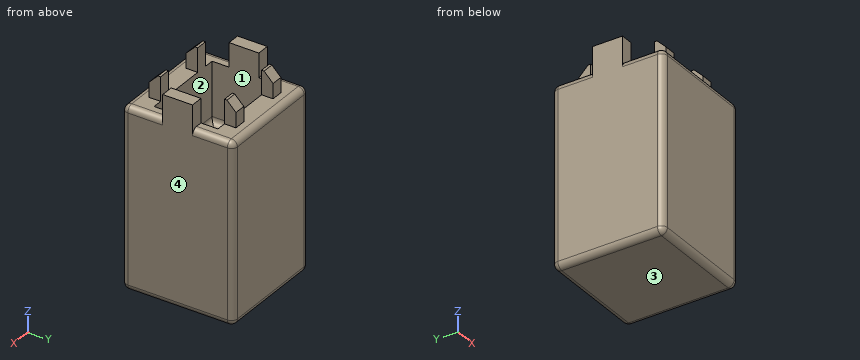
Autodesk Fusion 360 part; units mm, degrees
sketch "Sketch1" plane through (0, 0, 0) normal (0, 0, 1) x (1, 0, 0)
  line L0 (0, 0) -> (18.62, 0)
  line L1 (18.62, 0) -> (18.62, 14.49)
  line L2 (18.62, 14.49) -> (0, 14.49)
  line L3 (0, 14.49) -> (0, 0)
  line L4 (9.31, 0) -> (9.31, 14.49)
  line L5 (0, 7.245) -> (18.62, 7.245)
  line L6 (2.1, 9.73) -> (-2.1, 9.73)
  line L7 (-2.1, 9.73) -> (-2.1, 4.76)
  line L8 (-2.1, 4.76) -> (2.1, 4.76)
  line L9 (2.1, 4.76) -> (2.1, 9.73)
  line L10 (2.1, 9.73) -> (-2.1, 4.76) construction
  line L11 (-2.1, 9.73) -> (2.1, 4.76) construction
  line L12 (3.72, 0) -> (3.72, 14.49)
  line L13 (3.72, 14.49) -> (5.66, 14.49)
  line L14 (5.66, 14.49) -> (5.66, 12.57)
  line L15 (5.66, 12.57) -> (3.72, 12.57)
  line L16 (3.72, 12.57) -> (3.72, 14.49)
  line L17 (5.66, 1.92) -> (3.72, 1.92)
  line L18 (3.72, 1.92) -> (3.72, 0)
  line L19 (5.66, 0) -> (5.66, 1.92)
  line L20 (16.52, 9.73) -> (20.72, 9.73)
  line L21 (16.52, 4.76) -> (16.52, 9.73)
  line L22 (20.72, 4.76) -> (16.52, 4.76)
  line L23 (12.96, 14.49) -> (12.96, 12.57)
  line L24 (12.96, 12.57) -> (14.9, 12.57)
  line L25 (14.9, 12.57) -> (14.9, 14.49)
  line L26 (12.96, 1.92) -> (14.9, 1.92)
  line L27 (12.96, 0) -> (12.96, 1.92)
  line L28 (14.9, 0) -> (14.9, 14.49)
  line L29 (3.72, 12.57) -> (14.9, 12.57)
  line L30 (14.9, 12.57) -> (14.9, 1.92)
  line L31 (14.9, 1.92) -> (3.72, 1.92)
  line L32 (3.72, 1.92) -> (3.72, 12.57)
  line L33 (2.1, 9.73) -> (3.72, 9.73)
  line L34 (3.72, 9.73) -> (3.72, 12.57)
  line L35 (3.72, 12.57) -> (2.1, 12.57)
  line L36 (2.1, 12.57) -> (2.1, 9.73)
  line L37 (2.1, 4.76) -> (3.72, 4.76)
  line L38 (3.72, 4.76) -> (3.72, 1.92)
  line L39 (3.72, 1.92) -> (2.1, 1.92)
  line L40 (2.1, 1.92) -> (2.1, 4.76)
  line L41 (14.9, 1.92) -> (16.52, 1.92)
  line L42 (16.52, 1.92) -> (16.52, 4.76)
  line L43 (16.52, 4.76) -> (14.9, 4.76)
  line L44 (14.9, 4.76) -> (14.9, 1.92)
  line L45 (16.52, 9.73) -> (14.9, 9.73)
  line L46 (14.9, 9.73) -> (14.9, 12.57)
  line L47 (14.9, 12.57) -> (16.52, 12.57)
  line L48 (16.52, 12.57) -> (16.52, 9.73)
  circle A0 centre (9.31, 7.245) radius 2.5
  line L49 (18.62, -2.065) -> (0, -2.065)
  line L50 (0, -2.065) -> (0, 16.555)
  line L51 (0, 16.555) -> (18.62, 16.555)
  line L52 (18.62, 16.555) -> (18.62, -2.065)
  line L53 (18.62, -2.065) -> (0, 16.555) construction
  line L54 (0, -2.065) -> (18.62, 16.555) construction
  point P0 (0, 7.245)
  point P1 (9.31, 7.245)
  dimension "d1" = 18.62
  dimension "d2" = 14.49
  dimension "d3" = 4.2
  dimension "d4" = 4.97
  dimension "d5" = -5.59
  dimension "d6" = 1.94
  dimension "d7" = 1.92
  dimension "d16" = 5
  dimension "d19" = 18.62
  dimension "d20" = 18.62
extrude "Extrude1" add sketch "Sketch1" along normal blind 34 contours L0 L12 L17 L18 L19 L31 | L3 L5 L8 L9 L50 | L3 L5 L6 L9 L50 | L0 L26 L27 L28 L31 | L1 L5 L21 L22 L52 | L2 L12 L13 L14 L15 L16 L29 | L1 L5 L20 L21 L52 | L2 L23 L24 L25 L28 L29 makes body 1 at (13.6067, 0, 22.6667) makes body 2 at (5.0133, 14.49, 22.6667) makes body 3 at (18.62, 6.4167, 11.3333) makes body 4 at (4.3667, 0, 22.6667) makes body 5 at (0, 8.0733, 11.3333) makes body 6 at (14.2533, 14.49, 22.6667)
extrude "Extrude4" add sketch "Sketch1" along normal blind 30 contours L0 L3 L8 L12 L18 L39 L40 L50 | L0 L4 L19 L31 | L0 L4 L27 L31 | L2 L3 L6 L12 L16 L35 L36 L50 | L0 L1 L22 L28 L41 L42 L52 | L2 L4 L14 L29 | L1 L2 L20 L25 L28 L47 L48 L52 | L2 L4 L23 L29 bodies 1 2 3 4 5 6
extrude "Extrude5" add sketch "Sketch1" along normal blind 20 contours L12 L32 L37 L38 L39 L40 | L4 L5 L12 L17 L31 L32 L38 A0 | L5 L9 L12 L32 L37 | L5 L9 L12 L32 L33 | L4 L5 L26 L28 L30 L31 L44 A0 | L4 L5 L12 L15 L29 L32 L34 A0 | L12 L32 L33 L34 L35 L36 | L4 L5 A0 | L4 L5 A0 | L4 L5 A0 | L28 L30 L41 L42 L43 L44 | L5 L21 L28 L30 L43 | L4 L5 A0 | L4 L5 L24 L28 L29 L30 L46 A0 | L5 L21 L28 L30 L45 | L28 L30 L45 L46 L47 L48 bodies 1
extrude "Extrude6" add sketch "Sketch1" along normal blind 30 contours L0 L49 L50 L52 | L2 L13 L50 L51 L52 bodies 1
fillet "Fillet1" radius 1 4 edges at (18.62, 16.555, 15) (0, 16.555, 15) (0, -2.065, 15) (18.62, -2.065, 15) on bodies 1
fillet "Fillet2" radius 1 10 edges at (18.62, 12.6425, 30) (18.3271, 16.2621, 30) (9.31, 16.555, 30) (0.2929, 16.2621, 30) (0, 12.6425, 30) (0, 1.8475, 30) (0.2929, -1.7721, 30) (9.31, -2.065, 30) (18.3271, -1.7721, 30) (18.62, 1.8475, 30) on bodies 1
chamfer "Chamfer1" distance 1.5 angle 45 1 edges at (4.69, 0, 34) on bodies 1
chamfer "Chamfer2" distance 1.5 angle 45 1 edges at (13.93, 0, 34) on bodies 1
chamfer "Chamfer3" distance 1.5 angle 45 2 edges at (4.69, 14.49, 34) (13.93, 14.49, 34) on bodies 1
fillet "Fillet3" radius 1 4 edges at (9.31, 1.92, 20) (16.52, 7.245, 20) (2.1, 7.245, 20) (9.31, 12.57, 20) on bodies 1
fillet "Fillet4" radius 1 8 edges at (0.2929, -1.7721, 0) (0, 7.245, 0) (0.2929, 16.2621, 0) (9.31, 16.555, 0) (18.3271, 16.2621, 0) (18.62, 7.245, 0) (18.3271, -1.7721, 0) (9.31, -2.065, 0) on bodies 1
scale "Scale1" factor 1.01 about (0, -1.065, 29) bodies 1
Source: CAD feature listing. Evaluate the final solid. Frame: model axes, mm. Face numbers are marked on the shaded views. Round coordinates to 2 decimals unless told otherwise and drop trailing zeros. Loops run counter-clockwise (first coordinate to the right, second up) from the corner with the lowest first, then second, coordinate; pieces in that order, holes last. Notation, with made-up numbers: (-8.75, 57.25) -> (10.25, 57.25) arc R26 ccw to (10.25, 87.25) -> close; hole circle Ø2 at (-17, -7). An arc over 180 degrees is marked (long way). Answer as a JSON object with one key per item and string values. Group by question number.
Q1. Section query C-C (x = 17.25). Output: boundary loops of the cut face in (y, z) (3 decimals), plus the area to 3 significant figures.
Q2. Contact query for flat-ended pins moving along their axis: P1, Ø1, axis at y = 14, z = 32, coming from the +X side; P2, Ø0.6, axis at x = 17.5, z = 32, coming from the -Y side; P3, Ø1, axis at y = 1, z = 32, coming from the -X side. Output: stop coordinate, or through.
Q3. Section query A-A (z = 28.5). Output: boundary loops of the cut face in (x, y) (3 decimals), plus the area to 3 significant figures.
Q4. Section query D-D (x = 11). Output: boundary loops of the cut face in (y, z) (3 decimals), plus the area to 3 significant figures.
Q5. Mould query, pull axis X, two halves, no side actions, for the marked faces 1, 2, 3 and 4. Classes: pulls with the +X half, pulls with the -X half, needs draft (parallel to the pull), parting line crosses it, or undercut.
Q6. Ray query, line 1 (X direction, y = 7, z = 32); line 2 (Z direction, x = 3.5, y = 3); line 3 (Z direction, x = 7.5, y = 13.25). Return the intervals inside material, ascending. Write a range as from..to.
Q7. Section query B-B (y = 10.5). Output: boundary loops of the cut face in (x, z), plus the area to 3 significant figures.
Completed:
{
 "1": {"outline": "(-2.075, 0.72) arc R1.01 ccw to (-1.065, -0.29) -> (15.721, -0.29) arc R1.01 ccw to (16.731, 0.72) -> (16.731, 29) arc R1.01 ccw to (15.721, 30.01) -> (9.838, 30.01) -> (9.838, 34.05) -> (4.818, 34.05) -> (4.818, 30.01) -> (-1.065, 30.01) arc R1.01 ccw to (-2.075, 29) -> close", "area": "589 mm²"},
 "2": {"P1": "x = 15.05", "P2": "y = 4.82", "P3": "x = 3.76"},
 "3": {"outline": "(0, -1.065) arc R1.01 ccw to (1.01, -2.075) -> (17.796, -2.075) arc R1.01 ccw to (18.806, -1.065) -> (18.806, 15.721) arc R1.01 ccw to (17.796, 16.731) -> (1.01, 16.731) arc R1.01 ccw to (0, 15.721) -> close; hole (2.121, 1.95) -> (16.685, 1.95) -> (16.685, 12.706) -> (2.121, 12.706) -> close", "area": "196 mm²"},
 "4": {"outline": "(-2.075, 0.72) arc R1.01 ccw to (-1.065, -0.29) -> (15.721, -0.29) arc R1.01 ccw to (16.731, 0.72) -> (16.731, 29) arc R1.01 ccw to (15.721, 30.01) -> (12.706, 30.01) -> (12.706, 20.92) arc R1.01 cw to (11.696, 19.91) -> (2.96, 19.91) arc R1.01 cw to (1.95, 20.92) -> (1.95, 30.01) -> (-1.065, 30.01) arc R1.01 ccw to (-2.075, 29) -> close", "area": "461 mm²"},
 "5": {"face 1": "undercut", "face 2": "undercut", "face 3": "needs draft", "face 4": "pulls with the +X half"},
 "6": {"line 1": "0..2.12, 16.69..18.81", "line 2": "-0.29..19.91", "line 3": "-0.29..30.01"},
 "7": {"outline": "(0, 0.72) arc R1.01 ccw to (1.01, -0.29) -> (17.8, -0.29) arc R1.01 ccw to (18.81, 0.72) -> (18.81, 29) arc R1.01 ccw to (17.8, 30.01) -> (16.69, 30.01) -> (16.69, 20.92) arc R1.01 cw to (15.68, 19.91) -> (3.13, 19.91) arc R1.01 cw to (2.12, 20.92) -> (2.12, 30.01) -> (1.01, 30.01) arc R1.01 ccw to (0, 29) -> close", "area": "422 mm²"}
}
